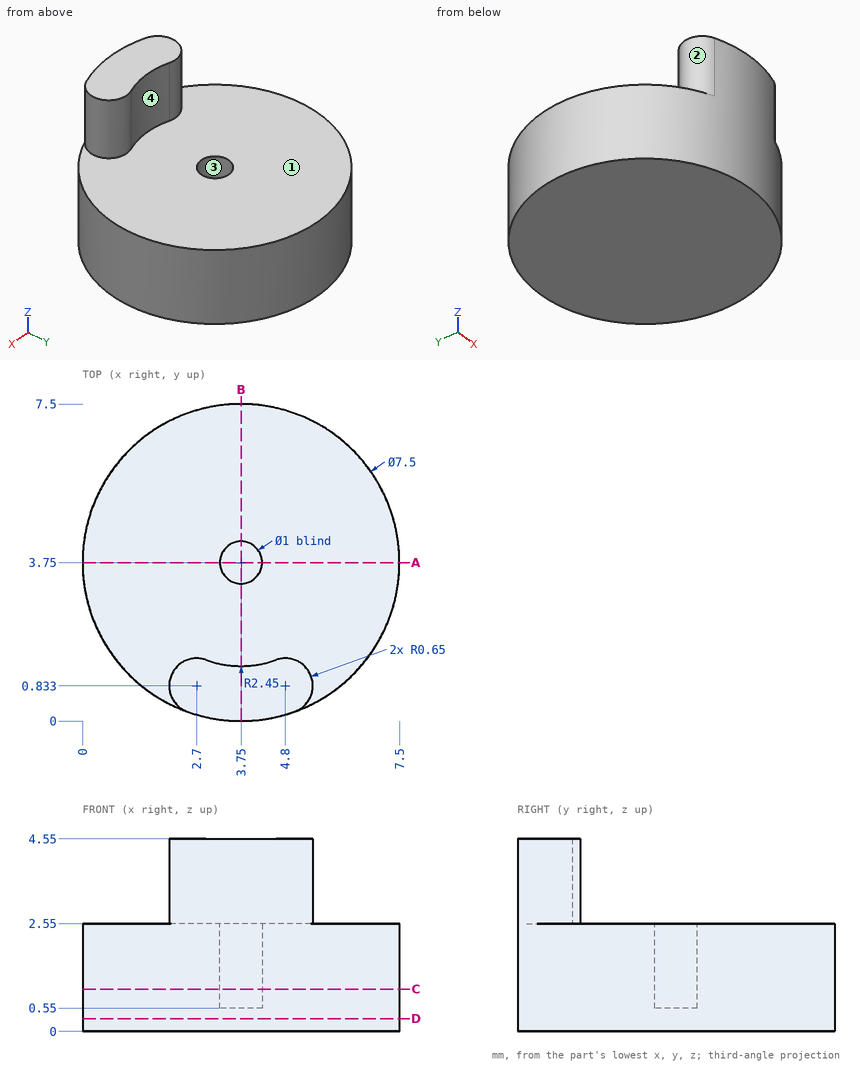
Part print with two shaded views. Sizes in mm from the minimum x, y, z corner. Round coordinates to 2 decimals unless told otherwise and drop trailing zeros. Order: outer loops, then holes, each group sorted by start corner. A loop starts at its lowest first (then second) coordinate and runs counter-clockwise, first axis right, second up. Notation, with made-up numbers: (-30, -24) - (-26, -24) arc R26 ccw to (-26, 2) - close; hole circle Ø6 at (12.25, 69). An arc over 180 degrees is marked (long way). Return JSON: item names as keys, results as strings.
(1) Cut at D-D (z = 0.3). Give the cut face in (x, y), then the cut area to 3 significant figures.
Answer key:
{"outline": "circle Ø7.5 at (3.75, 3.75)", "area": "44.2 mm^2"}
(2) Pin check, flat tip, straight feed: pin 1 Ø3 at (x, y) = (2, 5.5) entering from +Z. Stop position of the tip, or through.
Answer key:
{"pin 1": "stops at z = 2.55"}
(3) Cut at B-B (x = 3.75). Give the cut face in (y, z).
Answer key:
{"outline": "(0, 0) - (7.5, 0) - (7.5, 2.55) - (4.25, 2.55) - (4.25, 0.55) - (3.25, 0.55) - (3.25, 2.55) - (1.3, 2.55) - (1.3, 4.55) - (0, 4.55) - close"}
(4) Wall check: probe 1 along Y at (x, z) = (3.75, 1.2); probe 2 along Z at (x, y) = (1, 1.5); probe 3 along Y at (x, z) = (4.5, 4) (1 decimal). Give the ranges that are in metal, low to high. Write a range as from..to.
Answer key:
{"probe 1": "y = 0..3.25, 4.25..7.5", "probe 2": "z = 0..2.55", "probe 3": "y = 0.1..1.4"}
(5) Pull direction Y, two halves, no side cores. Call the marked faces 1, 2, 3 and 4: +Y half, -Y half, draft (parallel to the pull), parting line (faces both ways), or undercut.
Answer key:
{"face 1": "draft", "face 2": "parting line", "face 3": "undercut", "face 4": "+Y half"}
(6) Cut at A-A (y = 3.75). Give the cut face in (x, z), then the cut area to 3 significant figures.
Answer key:
{"outline": "(0, 0) - (7.5, 0) - (7.5, 2.55) - (4.25, 2.55) - (4.25, 0.55) - (3.25, 0.55) - (3.25, 2.55) - (0, 2.55) - close", "area": "17.1 mm^2"}
(7) Cut at C-C (z = 1). Give the cut face in (x, y).
Answer key:
{"outline": "circle Ø7.5 at (3.75, 3.75); hole circle Ø1 at (3.75, 3.75)"}
